from build123d import *

# Parameters (mm, degrees)
SKETCH_1_R      = 1.5
EXTRUDE_1_DEPTH = 3


with BuildPart() as part:
    # 草圖1 → 填料-伸長1 (new body)
    with BuildSketch(Plane(origin=(0, 3, 0), x_dir=(1, 0, 0), z_dir=(0, 1, 0))):
        with BuildLine():
            Line((-60, 57), (-60, -57))
            ThreePointArc((-60, -57), (-59.121320344, -59.121320344), (-57, -60))
            Line((-57, -60), (57, -60))
            ThreePointArc((57, -60), (59.121320344, -59.121320344), (60, -57))
            Line((60, -57), (60, 57))
            ThreePointArc((60, 57), (59.121320344, 59.121320344), (57, 60))
            Line((57, 60), (-57, 60))
            ThreePointArc((-57, 60), (-59.121320344, 59.121320344), (-60, 57))
        make_face()
        with Locations((-17.035, 50.6)):
            Circle(SKETCH_1_R, mode=Mode.SUBTRACT)
        with Locations((44.685, 50.6)):
            Circle(SKETCH_1_R, mode=Mode.SUBTRACT)
        with Locations((44.685, -26)):
            Circle(SKETCH_1_R, mode=Mode.SUBTRACT)
        with Locations((-17.035, -26)):
            Circle(SKETCH_1_R, mode=Mode.SUBTRACT)
        with Locations((52.5, -52.5)):
            Circle(SKETCH_1_R, mode=Mode.SUBTRACT)
        with Locations((-52.5, 52.5)):
            Circle(SKETCH_1_R, mode=Mode.SUBTRACT)
        with Locations((52.5, 52.5)):
            Circle(SKETCH_1_R, mode=Mode.SUBTRACT)
        with Locations((-52.5, -52.5)):
            Circle(SKETCH_1_R, mode=Mode.SUBTRACT)
        Polygon((-48, -21), (-48, 45.6), (-43, 50.6), (-26.535, 50.6), (-21.535, 45.6), (-21.535, -21), (-26.535, -26), (-43, -26), align=None, mode=Mode.SUBTRACT)
        Polygon((-17.035, -43), (-17.035, -35.5), (-12.035, -30.5), (39.685, -30.5), (44.685, -35.5), (44.685, -43), (39.685, -48), (-12.035, -48), align=None, mode=Mode.SUBTRACT)
        Polygon((-48, -43), (-48, -35.5), (-43, -30.5), (-26.535, -30.5), (-21.535, -35.5), (-21.535, -43), (-26.535, -48), (-43, -48), align=None, mode=Mode.SUBTRACT)
        Polygon((-7.035, 50.6), (34.685, 50.6), (44.685, 40.6), (44.685, -16), (34.685, -26), (-7.035, -26), (-17.035, -16), (-17.035, 40.6), align=None, mode=Mode.SUBTRACT)
    extrude(amount=-EXTRUDE_1_DEPTH)


solid = part.part
Geometry: final body of the model. Coordinates: model frame, mm. Give positions to 0.01 mm unless a question says otherwise; leave off trailing zeros. Loops run counter-clockwise (first coordinate to the right, second up) from the corner with the lowest first, then second, coordinate; pieces in that order, holes last. Notation, with made-up numbers: M 30.25,-33 L 64.25,-33 A11 cw 64.25,-20 Z; hole C 48,42.25 d7. An arc over 180 degrees is marked long. Put each result on its own line as item: value. Start each with the question number.
1) Pull-direction query (X, two-part tool) for faces 1 (the cylindrical face through (-53.7, 1.5, -51.6)), 2 (the cylindrical face through (59.1, 1.52, 59.14)), 3 (the flat face through (-35, 2, 26)); classes: pulls with the +X half, pulls with the -X half, needs draft (parallel to the pull), parting line crosses it, or undercut.
2) Cut plane C-C (y = 0.9). Give the number of separate pieces and of enclosed holes in the cut face, then the cut area to 3 significant figures.
3) Contact query for a flat-ended pin moving along its axis: pin 1 (1.8 mm diameter, centred on x = 44.685, z = 26, fed in from -Y). Output: stop coordinate, or through.
4) Cut plane B-B (x = -3). Output: boundary loops of the cut face in (y, z), then the cut area to 3 significant figures.
5) Cut plane A-A (z = 52.5). Output: boundary loops of the cut face in (x, y).
6) Ray query, line 1 along Z through (x, y) = (-52.5, 2.05); line 2 along Z through (x, y) = (33, 0.15); line 3 along X through (y, z) = (0.95, -16.5) (3 decimals). Return the intervals inside material, ascending.
Verdict:
1. face 1: undercut
1. face 2: pulls with the +X half
1. face 3: undercut
2. separate pieces: 1
2. enclosed holes: 12
2. area: 6,390 mm2
3. pin 1: through
4. outline: M 0,-60 L 3,-60 L 3,-50.6 L 0,-50.6 Z; M 0,26 L 3,26 L 3,30.5 L 0,30.5 Z; M 0,48 L 3,48 L 3,60 L 0,60 Z
4. area: 77.7 mm2
5. outline: M -60,0 L -54,0 L -54,3 L -60,3 Z; M -51,0 L 51,0 L 51,3 L -51,3 Z; M 54,0 L 60,0 L 60,3 L 54,3 Z
6. line 1: -60 to -54, -51 to 51, 54 to 60
6. line 2: -60 to -50.6, 26 to 30.5, 48 to 60
6. line 3: -60 to -48, -21.535 to -17.035, 44.685 to 60
